Verification items for this drawing (mm, ordinates from the low corner). Round coordinates to 2 decimals unless told otherwise and drop trailing zeros. Order: outer loops, then holes, each group sorted by start corner. A loop starts at its lowest first (then second) coordinate and runs counter-clockwise, first axis right, second up.
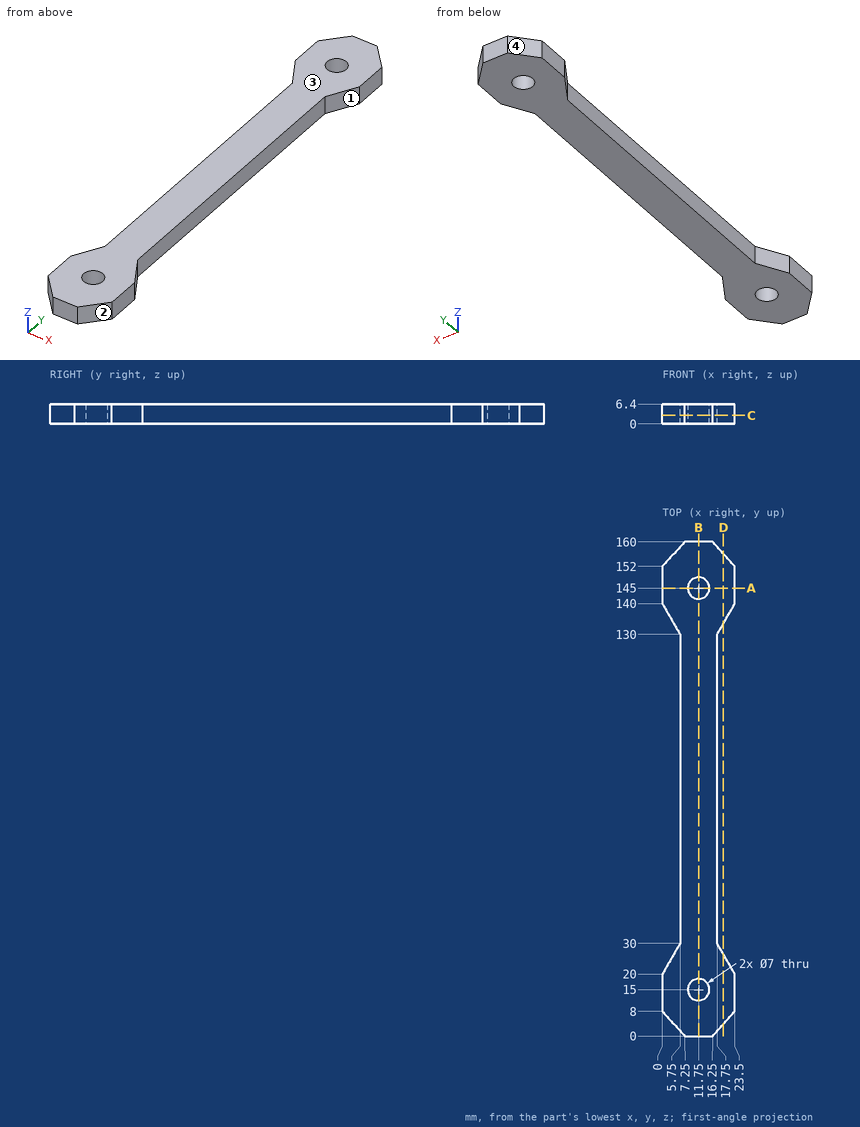
Item 1: Sectioned sample at C-C (z = 2.75). Record the cut outline in (x, y).
Answer:
outline: (0, 8) - (7.25, 0) - (16.25, 0) - (23.5, 8) - (23.5, 20) - (17.75, 30) - (17.75, 130) - (23.5, 140) - (23.5, 152) - (16.25, 160) - (7.25, 160) - (0, 152) - (0, 140) - (5.75, 130) - (5.75, 30) - (0, 20) - close; hole circle Ø7 at (11.75, 15); hole circle Ø7 at (11.75, 145)
Item 2: Sectioned sample at A-A (y = 145). Record the cut outline in (x, z).
Answer:
outline: (0, 0) - (8.25, 0) - (8.25, 6.4) - (0, 6.4) - close; (15.25, 0) - (23.5, 0) - (23.5, 6.4) - (15.25, 6.4) - close
Item 3: Sectioned sample at B-B (x = 11.75). Record the cut outline in (y, z).
Answer:
outline: (0, 0) - (11.5, 0) - (11.5, 6.4) - (0, 6.4) - close; (18.5, 0) - (141.5, 0) - (141.5, 6.4) - (18.5, 6.4) - close; (148.5, 0) - (160, 0) - (160, 6.4) - (148.5, 6.4) - close
Item 4: Release check for a two-part mould opening along Y. For the marked faces 1, 2, 3 and 4 record: released by +Y, released by -Y, zero draft, split by the parting line, or undercut.
Answer:
face 1: undercut
face 2: released by -Y
face 3: zero draft
face 4: released by +Y
Item 5: Go/stop test with flat-tipped pins: P1, Ø3, axis at y = 101.5, z = 3.5, coming from the -X side; P2, Ø2, axis at y = 129.5, z = 5.5, coming from the -X side; P3, Ø1, axis at x = 17, y = 136.5, coming from the -Z side; P4, Ø3, axis at y = 81.5, z = 2.5, coming from the +X side. Record where each tip stops, or that it passes through.
Answer:
P1: stops at x = 5.75
P2: stops at x = 5.46
P3: stops at z = 0
P4: stops at x = 17.75
Item 6: Sectioned sample at D-D (x = 19.75). Record the cut outline in (y, z), and give its area (3 significant figures).
Answer:
outline: (3.86, 0) - (26.52, 0) - (26.52, 6.4) - (3.86, 6.4) - close; (133.48, 0) - (156.14, 0) - (156.14, 6.4) - (133.48, 6.4) - close
area: 290 mm2
Item 7: Scan lines: line 1 along Y through (x, z) = (11.75, 4.5); line 2 along X through (y, z) = (145, 2.75); line 3 along Y through (x, z) = (10, 4). Record each from-to range of solid material in increasing order.
Answer:
line 1: y = 0 to 11.5, 18.5 to 141.5, 148.5 to 160
line 2: x = 0 to 8.25, 15.25 to 23.5
line 3: y = 0 to 11.97, 18.03 to 141.97, 148.03 to 160
